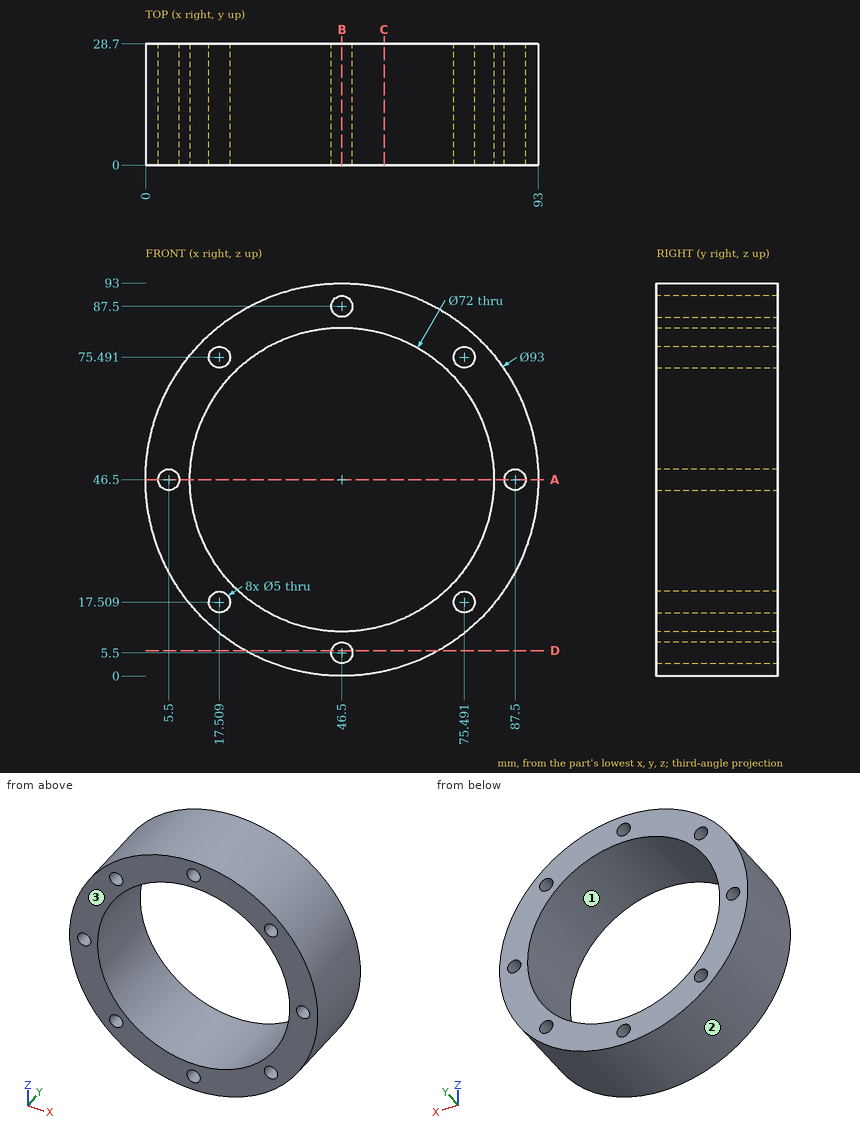
The drawing under review shows one solid part. Ordinate dimensions are in mm from its lowest x, y, z. Round coordinates to 2 decimals unless told otherwise and drop trailing zeros. Order: outer loops, then holes, each group sorted by start corner. A loop starts at its lowest first (then second) coordinate and runs counter-clockwise, first axis right, second up. Notation, with made-up numbers: (-36, -20.75) -> (6, -20.75) arc R9 ccw to (6, -15.75) -> close; hole circle Ø11 at (-37.75, 2.25). An arc over 180 degrees is marked (long way). Return JSON: item names as keys, results as strings.
1. Take a section at A-A (z = 46.5). Write out the cut boundary in (x, y).
Answer block:
{"outline": "(0, 0) -> (3, 0) -> (3, 28.7) -> (0, 28.7) -> close; (8, 0) -> (10.5, 0) -> (10.5, 28.7) -> (8, 28.7) -> close; (82.5, 0) -> (85, 0) -> (85, 28.7) -> (82.5, 28.7) -> close; (90, 0) -> (93, 0) -> (93, 28.7) -> (90, 28.7) -> close"}
2. Take a section at B-B (x = 46.5). Write out the cut boundary in (y, z), then the cut area to 3 significant figures.
Answer block:
{"outline": "(0, 0) -> (28.7, 0) -> (28.7, 3) -> (0, 3) -> close; (0, 8) -> (28.7, 8) -> (28.7, 10.5) -> (0, 10.5) -> close; (0, 82.5) -> (28.7, 82.5) -> (28.7, 85) -> (0, 85) -> close; (0, 90) -> (28.7, 90) -> (28.7, 93) -> (0, 93) -> close", "area": "316 mm²"}
3. Take a section at D-D (z = 6). Write out the cut boundary in (x, y).
Answer block:
{"outline": "(23.65, 0) -> (44.05, 0) -> (44.05, 28.7) -> (23.65, 28.7) -> close; (48.95, 0) -> (69.35, 0) -> (69.35, 28.7) -> (48.95, 28.7) -> close"}
4. The part is to be moulded in two halves that separate along Z. For the marked faces 1, 2 and 3, say which applies: +Z half, -Z half, draft (parallel to the pull), parting line (faces both ways), or undercut.
Answer block:
{"face 1": "undercut", "face 2": "parting line", "face 3": "draft"}
5. For L1, parallel to X at y = 11.25, z = 46.5; L2, parallel to Z at x = 45.5, y = 12.75 (1 decimal); L3, parallel to X at y = 20.5, z = 35.5, list the stretches that pass through material, from the lowest coordinate up. Write a range as [from, to].
Answer block:
{"L1": "x = [0, 3], [8, 10.5], [82.5, 85], [90, 93]", "L2": "z = [0, 3.2], [7.8, 10.5], [82.5, 85.2], [89.8, 93]", "L3": "x = [1.32, 12.22], [80.78, 91.68]"}
6. Take a section at C-C (x = 56.5). Write out the cut boundary in (y, z).
Answer block:
{"outline": "(0, 1.09) -> (28.7, 1.09) -> (28.7, 11.92) -> (0, 11.92) -> close; (0, 81.08) -> (28.7, 81.08) -> (28.7, 91.91) -> (0, 91.91) -> close"}
7. Insertion check: P1, Ø6.5, axis at x = 75.49, z = 17.51, coming from the +Y side; P2, Ø6, axis at x = 51.5, y = 17.5, coming from the +Z side; P3, Ø5, axis at y = 23.5, z = 46, coming from the -X side; P4, Ø3, axis at y = 4.5, z = 40.5, coming from the +X side. Each pin has a flat end and moves straight along its axis. Give the tip position at first contact, or say it passes through.
Answer block:
{"P1": "stops at y = 28.7", "P2": "stops at z = 92.96", "P3": "stops at x = 0", "P4": "stops at x = 92.78"}
